Autodesk Inventor part; units mm, degrees
ref_plane "YZ Plane" through (0, 0, 0) normal (1, 0, 0) x (0, 1, 0)
ref_plane "XZ Plane" through (0, 0, 0) normal (0, 1, 0) x (-1, 0, 0)
ref_plane "XY Plane" through (0, 0, 0) normal (0, 0, 1) x (1, 0, 0)
sketch "Sketch1" plane through (0, 0, 0) normal (0, 0, 1) x (1, 0, 0)
  circle A0 centre (0, 0) radius 5.5
  circle A1 centre (0, 0) radius 2.5
  line L0 (0, 0) -> (0, 5.5) construction
  line L1 (0, 0) -> (-3.8891, 3.8891)
  line L2 (0, 0) -> (3.8891, 3.8891)
  point P0 (1.7678, 1.7678)
  point P1 (-1.7678, 1.7678)
  dimension "d0" = 5
  dimension "d1" = 3
  dimension "d2" = 45
  dimension "d3" = 45
extrude "Extrusion1" add sketch "Sketch1" along normal mid plane 8 contours A0 L1 A1 L2 picked at (-3.4581, 2.8281)
sketch "Sketch2" plane through (0, 0, 0) normal (0, 0, 1) x (1, 0, 0)
  arc A0 (-3.8891, 3.8891) -> (3.8891, 3.8891) centre (0, 0) ccw construction
  line L0 (4.899, 2.5) -> (42.899, 2.5)
  line L1 (42.899, 2.5) -> (42.899, -2.5)
  line L2 (42.899, -2.5) -> (4.899, -2.5)
  line L3 (4.899, -2.5) -> (4.899, 2.5)
  line L4 (0, 0) -> (42.899, 0)
  point P0 (4.899, 0)
  dimension "d6" = 38
  dimension "d7" = 5
revolve "Revolution1" add sketch "Sketch2" angle 360 about axis through (0, 0, 0) along (1, 0, 0) contours L0 L1 L4 L3
chamfer "Chamfer1" distance 2 angle 45 1 edges at (42.899, -2.5, 0)
fillet "Fillet3" radius 1 4 edges at (-3.8891, 3.8891, 0) (-1.7678, 1.7678, 0) (3.8891, 3.8891, 0) (1.7678, 1.7678, 0)
properties part number "Apple_logo_Black_Part2"
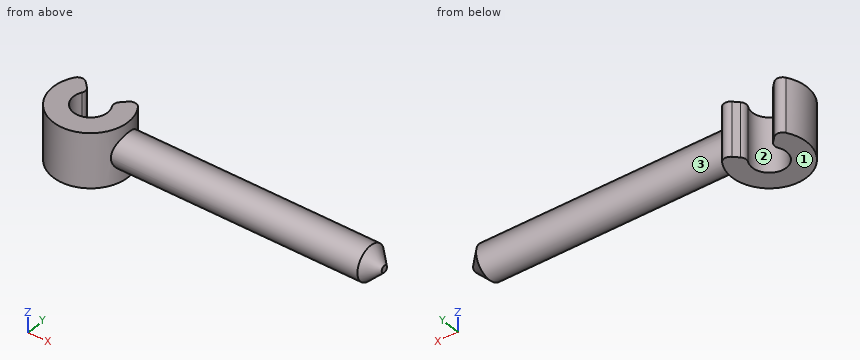
The listing builds one solid part. Answer for the finished solid, in the listing's coordinates (mm). Face numbers are marked on the shaded views. Coordinates: 2 decimals unless noted, no trailing zeros. Write each loop counter-clockwise with the first axis right and the second up, starting at its lowest first coordinate (ties: lowest second). Pieces come first, ordered by that corner, then holes. Notation, with made-up numbers: (-37, 38.5) - (-24, 38.5) arc R12 ccw to (-24, 49.5) - close; hole circle Ø9 at (57.25, 55). An arc over 180 degrees is marked (long way). Put each result on its own line as item: value.
1. Flat-ended cylindrical pins translate along their axes: pin 1 Ø3 at (x, y) = (22, 2) entering from +Z; pin 2 Ø1.5 at (x, z) = (28.5, -2) entering from +Y; pin 3 Ø2 at (x, y) = (12.5, 2.5) entering from +Z. Find the tip coordinate at first contact, or state that the pin passes through.
Answer sheet:
pin 1: stops at z = 2.45
pin 2: stops at y = 2.17
pin 3: stops at z = 2
2. The part is cut by section B-B on x = 9.5. Give the vertices of the cut face in (y, z).
Answer sheet:
outline: circle Ø5 at (0, 0)
3. Determine the mould class of the marked faces 1, 2 and 3 for opening direction Y: pulls with the +Y half, pulls with the -Y half, needs draft (parallel to the pull), parting line crosses it, or undercut.
Answer sheet:
face 1: needs draft
face 2: undercut
face 3: parting line crosses it
4. The part is cut by section A-A on y = 0. Give the vertices of the cut face in (x, z).
Answer sheet:
outline: (-5.5, -4) - (-2.5, -4) - (-2.5, 4) - (-5.5, 4) - close; (2.5, -4) - (5.5, -4) - (5.5, -2.5) - (40.9, -2.5) - (42.9, -0.5) - (42.9, 0.5) - (40.9, 2.5) - (5.5, 2.5) - (5.5, 4) - (2.5, 4) - close
5. Find the intervals of material crossed by line 1 along X through (y, z) = (0, -0.25); line 2 along X through (y, z) = (0, -1); line 3 along Z through (x, y) = (19, -1.5), in increasing order. Write a range as from..to.
Answer sheet:
line 1: x = -5.5..-2.5, 2.5..42.9
line 2: x = -5.5..-2.5, 2.5..42.4
line 3: z = -2..2
6. The part is cut by section C-C on x = 0. Give the vertices of the cut face in (y, z).
Answer sheet:
outline: (-5.5, -4) - (-2.5, -4) - (-2.5, 4) - (-5.5, 4) - close
